Build history of the part. All positions in model axes, mm. A direction names the side the tool comes from. Round coordinates to 2 decimals unless told otherwise and drop trailing zeros. Loops run counter-clockwise (first coordinate to the right, second up) from the corner with the lowest first, then second, coordinate; pieces in that order, holes last. Notation, with made-up numbers: (27.5, 68.5) - (57.5, 68.5) arc R23 ccw to (57.5, 86.5) - close; hole circle Ø6 at (-9, 16). An arc over 180 degrees is marked (long way). Use a Markdown table: item, result.
from build123d import *

# Parameters (mm, degrees)
SKETCH1_R           = 7.5
BOSS_EXTRUDE1_DEPTH = 204.47
SKETCH2_R           = 10
BOSS_EXTRUDE2_DEPTH = 5
SKETCH3_R           = 10
BOSS_EXTRUDE3_DEPTH = 2.5
SKETCH4_R           = 10
BOSS_EXTRUDE4_DEPTH = 2.5


with BuildPart() as part:
    # Sketch1 → Boss-Extrude1 (new body, symmetric)
    with BuildSketch(Plane(origin=(0, 0, 0), x_dir=(0, 0, -1), z_dir=(1, 0, 0))):
        Circle(SKETCH1_R)
    extrude(amount=BOSS_EXTRUDE1_DEPTH, both=True)


with BuildPart() as body_2:
    # Sketch2 → Boss-Extrude2 (new body)
    with BuildSketch(Plane(origin=(204.47, 0, 0), x_dir=(0, 0, -1), z_dir=(1, 0, 0))):
        Circle(SKETCH2_R)
    extrude(amount=BOSS_EXTRUDE2_DEPTH)


with BuildPart() as body_3:
    # Mirror1: mirrored copy
    add(body_2.part.mirror(Plane(origin=(0, 0, 0), x_dir=(0, 0, 1), z_dir=(1, 0, 0))))

    # Combine1: union body 2, part
    add(body_2.part)
    add(part.part)

    # Sketch3 → Boss-Extrude3 (add, symmetric)
    with BuildSketch(Plane(origin=(-68.469999966, 0, 0), x_dir=(0, 0, -1), z_dir=(1, 0, 0))):
        Circle(SKETCH3_R)
    extrude(amount=BOSS_EXTRUDE3_DEPTH, both=True)

    # Sketch4 → Boss-Extrude4 (add, symmetric)
    with BuildSketch(Plane.ZY.offset(-68.469999966)):
        Circle(SKETCH4_R)
    extrude(amount=BOSS_EXTRUDE4_DEPTH, both=True)


solid = body_3.part
Q1. Probe line 1 (X direction, y = 7.75, z = 6); line 2 (Z direction, x = 32, y = 1); line 3 (Y direction, x = -182.5, z = 0.5). List the from-to ranges inside material, lowest first.
Results found:
| item | result |
|---|---|
| line 1 | x = -209.47 to -204.47, -70.97 to -65.97, 65.97 to 70.97, 204.47 to 209.47 |
| line 2 | z = -7.43 to 7.43 |
| line 3 | y = -7.48 to 7.48 |
Q2. Which spindle directions (+Z, -Z, +X, -X, +Y, -Y) get a long thin tool onto all of the face, cutting with end or side? Do faces 1 (the face through (0.924, 0.33, 7.493)), 2 (the face through (68.43, -9.76, -2.17)). Say none if no direction does.
Results found:
| item | result |
|---|---|
| face 1 | none |
| face 2 | +X, -X |
Q3. Cut at A-A, the plane z = 0. List the corners of the cut face in (x, y).
Results found:
| item | result |
|---|---|
| outline | (-209.47, -10) - (-204.47, -10) - (-204.47, -7.5) - (-70.97, -7.5) - (-70.97, -10) - (-65.97, -10) - (-65.97, -7.5) - (65.97, -7.5) - (65.97, -10) - (70.97, -10) - (70.97, -7.5) - (204.47, -7.5) - (204.47, -10) - (209.47, -10) - (209.47, 10) - (204.47, 10) - (204.47, 7.5) - (70.97, 7.5) - (70.97, 10) - (65.97, 10) - (65.97, 7.5) - (-65.97, 7.5) - (-65.97, 10) - (-70.97, 10) - (-70.97, 7.5) - (-204.47, 7.5) - (-204.47, 10) - (-209.47, 10) - close |
Q4. Pull direction X, two halves, no side cores. Call faces 3 (the face through (65.97, 7, 4)), 4 (the face through (-209.47, 0, 0)), 5 (the face through (206.94, -9.76, 2.17)): pulls with the +X half, pulls with the -X half, needs draft (parallel to the pull), parting line crosses it, or undercut.
Results found:
| item | result |
|---|---|
| face 3 | undercut |
| face 4 | pulls with the -X half |
| face 5 | needs draft |
Q5. Cut at C-C, the plane x = -10. List the corners of the cut face in (y, z).
Results found:
| item | result |
|---|---|
| outline | circle Ø15 at (0, 0) |
Q6. Drop flat-ended pins along their axis: pin 1 (4 mm diameter, centred on x = 112.5, z = -7.5, fed in from +Y); pin 2 (6 mm diameter, centred on x = -17, y = 5, fed in from -Z); pin 3 (2 mm diameter, centred on x = -121, y = 7.5, fed in from -Z). Give the stop position or say it passes through.
Results found:
| item | result |
|---|---|
| pin 1 | stops at y = 5.1 |
| pin 2 | stops at z = -7.23 |
| pin 3 | stops at z = -3.74 |
